Part model, mm, in its own coordinate system. Coordinates: 2 decimals unless noted, no trailing zeros. Order: outer loops, then holes, each group sorted by start corner. A loop starts at its lowest first (then second) coordinate and runs counter-clockwise, first axis right, second up. Notation, with made-up numbers: (27, 89.5) - (48, 89.5) arc R31 ccw to (48, 120.5) - close; hole circle Ø1 at (-17, 50). An arc over 180 degrees is marked (long way). Use a Markdown table: item, result. Add a question column.
1) Wall check: L1, parallel to X at y = 0.65, z = -117.5; L2, parallel to X at y = -0.1, z = -52.5; L3, parallel to X at y = -0.4, z = -155.5. Give the ranges that are in metal, low to high. Write a range as [from, to].
2) Drop flat-ended pins along their axis: P1, Ø8, axis at x = -38.5, z = -114.5, coming from the -Y side; P2, Ø1, axis at x = -45.5, y = 0.5, coming from the -Z side. Give the stop position or say it passes through.
3) Saw through at B-B on y = 0. List the corners of the cut face in (x, z) (1 decimal).
4) Saw through at A-A on z = -34. List the corners of the cut face in (x, y) (1 decimal), then the cut area to 3 significant figures.
```python
from build123d import *

# Parameters (mm, degrees)
SKETCH2_R = 1.5875
SKETCH3_R = 1.5875


with BuildPart() as part:
    # Sweep1: sweep along a path in Sketch1
    with BuildLine(Plane(origin=(0, 0, 0), x_dir=(1, 0, 0), z_dir=(0, 1, 0))) as sweep1_path:
        Line((0, 0), (0, 73.025))
        Line((0, 73.025), (76.2, 149.225))
        Line((76.2, 149.225), (76.2, 174.625))
    # Sketch2 → Sweep1 (sweep)
    with BuildSketch(Plane.XY):
        Circle(SKETCH2_R)
    sweep(path=sweep1_path.line, transition=Transition.RIGHT)

    # Sweep4: sweep along a path in Sketch4
    with BuildLine(Plane(origin=(0, 0, 0), x_dir=(1, 0, 0), z_dir=(0, 1, 0))) as sweep4_path:
        Line((-76.2, 174.625), (-76.2, 149.225))
        Line((-76.2, 149.225), (0, 73.025))
    # Sketch3 → Sweep4 (sweep)
    with BuildSketch(Plane(origin=(-76.2, 0, -174.625), x_dir=(1, 0, 0), z_dir=(0, 0, 1))):
        Circle(SKETCH3_R)
    sweep(path=sweep4_path.line, transition=Transition.RIGHT)


solid = part.part
```
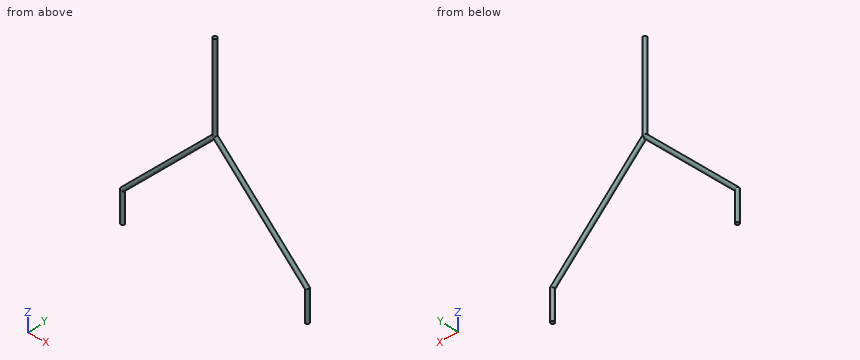
Results are:
| question | item | result |
|---|---|---|
| 1 | L1 | [-46.52, -42.43], [42.43, 46.52] |
| 1 | L2 | [-1.58, 1.58] |
| 1 | L3 | [-77.74, -74.66], [74.66, 77.74] |
| 2 | P1 | y = -1.59 |
| 2 | P2 | z = -121.19 |
| 3 | outline | (-77.8, -174.6) - (-74.6, -174.6) - (-74.6, -149.9) - (0, -75.3) - (74.6, -149.9) - (74.6, -174.6) - (77.8, -174.6) - (77.8, -148.6) - (1.6, -72.4) - (1.6, 0) - (-1.6, 0) - (-1.6, -72.4) - (-77.8, -148.6) - close |
| 4 | outline | circle Ø3.2 at (0, 0) |
| 4 | area | 7.92 mm2 |
